Geometry check sheet. Reference: the model listing, model coordinates, mm. A direction names the side the tool comes from. Coordinates: 2 decimals unless noted, no trailing zeros. Loops run counter-clockwise (first coordinate to the right, second up) from the corner with the lowest first, then second, coordinate; pieces in that order, holes last.
from build123d import *

# Parameters (mm, degrees)
EXTRUDE_START                = 29.8
SKETCH_1_W                   = 11.5
SKETCH_1_H                   = 21.4
EXTRUDE_21_4X11_5_20_6_DEPTH = 20.6
EXTRUDE_START_2              = 36
SKETCH_2_W                   = 11.5
SKETCH_2_H                   = 30
SKETCH_2_R                   = 1
EXTRUDE_30_26_4_2_2_DEPTH    = 2
EXTRUDE_START_3              = 27
SKETCH_3_R                   = 2.5
EXTRUDE_5_2_8_DEPTH          = 2.8


with BuildPart() as part:
    # 草图1 → 机身21.4x11.5_总高20.6 (new body)
    with BuildSketch(Plane(origin=(0, 0, 0), x_dir=(0, 0, -1), z_dir=(1, 0, 0)).offset(EXTRUDE_START)):
        with Locations((3.5, -4.95)):
            Rectangle(SKETCH_1_W, SKETCH_1_H)
    extrude(amount=EXTRUDE_21_4X11_5_20_6_DEPTH)

    # 草图2 → 安装耳30_孔距26.4_孔径2_耳厚暂定2 (add)
    with BuildSketch(Plane(origin=(0, 0, 0), x_dir=(0, 0, -1), z_dir=(1, 0, 0)).offset(EXTRUDE_START_2)):
        with Locations((3.5, -4.95)):
            Rectangle(SKETCH_2_W, SKETCH_2_H)
        with Locations((3.5, -18.15)):
            Circle(SKETCH_2_R, mode=Mode.SUBTRACT)
        with Locations((3.5, 8.25)):
            Circle(SKETCH_2_R, mode=Mode.SUBTRACT)
    extrude(amount=EXTRUDE_30_26_4_2_2_DEPTH)

    # 草图3 → 输出齿轴简化_直径5高2.8待实测 (add)
    with BuildSketch(Plane(origin=(0, 0, 0), x_dir=(0, 0, -1), z_dir=(1, 0, 0)).offset(EXTRUDE_START_3)):
        with Locations((3.5, 0)):
            Circle(SKETCH_3_R)
    extrude(amount=EXTRUDE_5_2_8_DEPTH)


solid = part.part
(1) Draft check along Y on faces 1 (the cylindrical face through (36.99, 9.24, -3.37)), 2 (the flat face through (36, -17, -3)), 3 (the cylindrical face through (36.99, -18.76, -2.71)), 4 (the cylindrical face through (28.38, 0.751, -5.885)). Enter one of: +Y half, -Y half, draft (parallel to the pull), parting line (faces both ways), or undercut.
Findings:
face 1: undercut
face 2: draft
face 3: undercut
face 4: parting line
(2) Scan lines: L1, parallel to Y at x = 37.25, z = -3.5; L2, parallel to X at y = -16.25, z = -4.5; L3, parallel to X at y = 3.5, z = 1. Record each from-to range of solid material in increasing order.
Findings:
L1: y = -19.95 to -19.15, -17.15 to 7.25, 9.25 to 10.05
L2: x = 36 to 38
L3: x = 29.8 to 50.4
(3) Sectioned sample at D-D on z = -7.75. Record the cut outline in (x, y), and give its area (3 significant figures).
Findings:
outline: (29.8, -15.65) - (36, -15.65) - (36, -19.95) - (38, -19.95) - (38, -15.65) - (50.4, -15.65) - (50.4, 5.75) - (38, 5.75) - (38, 10.05) - (36, 10.05) - (36, 5.75) - (29.8, 5.75) - close
area: 458 mm2
(4) Sectioned sample at A-A on z = -3.5. Record the cut outline in (x, y).
Findings:
outline: (27, -2.5) - (29.8, -2.5) - (29.8, -15.65) - (36, -15.65) - (36, -17.15) - (38, -17.15) - (38, -15.65) - (50.4, -15.65) - (50.4, 5.75) - (38, 5.75) - (38, 7.25) - (36, 7.25) - (36, 5.75) - (29.8, 5.75) - (29.8, 2.5) - (27, 2.5) - close; (36, -19.95) - (38, -19.95) - (38, -19.15) - (36, -19.15) - close; (36, 9.25) - (38, 9.25) - (38, 10.05) - (36, 10.05) - close
(5) Gauge pin test, flat ends, axial feed: pin 1 Ø2 at (y, z) = (-18, -2) entering from -X; pin 2 Ø1 at (y, z) = (-1, -0.5) entering from -X; pin 3 Ø4.5 at (y, z) = (-18.5, -5.5) entering from +X. Record the tip position at first contact, or that the pin passes through.
Findings:
pin 1: stops at x = 36
pin 2: stops at x = 29.8
pin 3: stops at x = 38
(6) Sectioned sample at C-C on x = 37. Record the cut outline in (y, z), and give its area (3 significant figures).
Findings:
outline: (-19.95, -9.25) - (10.05, -9.25) - (10.05, 2.25) - (-19.95, 2.25) - close; hole circle Ø2 at (-18.15, -3.5); hole circle Ø2 at (8.25, -3.5)
area: 339 mm2
(7) Access from +Z, -Z, +X, -X, +Y, -Y to the whole of each face (thin tool, end or side, straight path). Record for faces 5 (the flat face through (36, 7, -3)), 6 (the flat face through (44, -15.65, -3)), 7 (the flat face through (33, -15.65, -3)), 8 (the flat face through (38, 7, -3)).
Findings:
face 5: +Z, -Z, -X, +Y
face 6: +Z, -Z, +X, -Y
face 7: +Z, -Z, -X, -Y
face 8: +Z, -Z, +X, +Y
(8) Sectioned sample at B-B on y = -18.15. Record the cut outline in (x, z), and give its area (3 significant figures).
Findings:
outline: (36, -9.25) - (38, -9.25) - (38, -4.5) - (36, -4.5) - close; (36, -2.5) - (38, -2.5) - (38, 2.25) - (36, 2.25) - close
area: 19.0 mm2
